Source: CAD feature listing. Evaluate the final solid. Frame: model axes, mm. Give positions to 0.01 mm unless a question says otherwise; leave off trailing zeros. Write each loop counter-clockwise with the first axis right and the second up, starting at its lowest first coordinate (ties: lowest second). Pieces come first, ordered by that corner, then holes. Notation, with made-up numbers: (83, 31.5) -> (104, 31.5) arc R9 cw to (104, 43.5) -> close; hole circle Ø2 at (17.5, -30). An arc over 180 degrees is marked (long way). Answer as a JSON object with one key per item and string values. Group by question number.
Item 1: Ray query, probe 1 along Y at (x, z) = (12.75, 1.45); probe 2 along X at (y, z) = (-2.5, 0.7); probe 3 along Y at (x, z) = (11.25, 2). Return the intervals inside material, ascending. Write a range as from..to.
Item 2: Section query C-C on x = 12.25. Return the cut outline in (y, z), plus the area to 3 significant figures.
Item 3: Section query A-A on z = 0.75. Return the cut outline in (x, y), plus the area to 3 significant figures.
Item 4: First-contact query: pin 1 Ø6 at (x, y) = (7, -2.5) entering from -Z; pin 2 Ø1.5 at (x, z) = (17.5, 1.5) entering from +Y. Flat tips, straight axial feed; report the tip coordinate or a pass-through.
Item 5: Section query B-B on y = -5. Return the cut outline in (x, z), plus the area to 3 significant figures.
Autodesk Inventor part; units mm, degrees
ref_plane "YZ Plane" through (0, 0, 0) normal (1, 0, 0) x (0, 1, 0)
ref_plane "XZ Plane" through (0, 0, 0) normal (0, 1, 0) x (-1, 0, 0)
ref_plane "XY Plane" through (0, 0, 0) normal (0, 0, 1) x (1, 0, 0)
sketch "草图2" plane through (0, 0, 0) normal (0, 0, 1) x (1, 0, 0)
  arc A0 (11.812, -10.0858) -> (14.4114, -9.0466) centre (12.5814, -8.2397) ccw
  arc A1 (11.812, -10.0858) -> (-0.838, -5.8193) centre (-25.1186, -98.698) ccw
  arc A2 (-3.01, -2.276) -> (-0.838, -5.8193) centre (-0.0792, -2.9169) ccw
  line L0 (-0.4446, 9.4555) -> (-3.01, -2.276)
  arc A3 (3.2323, 11.7204) -> (-0.4446, 9.4555) centre (2.4862, 8.8147) ccw
  arc A4 (19.0048, 6.4168) -> (3.2323, 11.7204) centre (-25.1186, -98.698) ccw
  arc A5 (20.0607, 3.7658) -> (19.0048, 6.4168) centre (18.2307, 4.5727) ccw
  line L1 (14.4114, -9.0466) -> (20.0607, 3.7658)
  arc A6 (19.9692, 3.8061) -> (18.9661, 6.3246) centre (18.2307, 4.5727) ccw
  arc A7 (18.9661, 6.3246) -> (3.2074, 11.6235) centre (-25.1186, -98.698) ccw
  arc A8 (3.2074, 11.6235) -> (-0.3469, 9.4342) centre (2.4862, 8.8147) ccw
  line L2 (-0.3469, 9.4342) -> (-2.9123, -2.2974)
  arc A9 (-2.9123, -2.2974) -> (-0.8127, -5.7226) centre (-0.0792, -2.9169) ccw
  arc A10 (11.8505, -9.9935) -> (-0.8127, -5.7226) centre (-25.1186, -98.698) ccw
  arc A11 (11.8505, -9.9935) -> (14.3199, -9.0062) centre (12.5814, -8.2397) ccw
  line L3 (14.3199, -9.0062) -> (19.9692, 3.8061)
  dimension "d2" = 0.1
extrude "拉伸1" add sketch "草图2" along normal blind 3 contours L3 A11 A10 A9 L2 A8 A7 A6
properties part number "斜板固定件"
Worked answers:
{
 "1": {"probe 1": "-10.13..8.72", "probe 2": "-2.95..17.19", "probe 3": "-9.75..9.24"},
 "2": {"outline": "(-10.11, 0) -> (8.9, 0) -> (8.9, 3) -> (-10.11, 3) -> close", "area": "57.0 mm^2"},
 "3": {"outline": "(-2.91, -2.3) arc R2.9 ccw to (-0.81, -5.72) arc R96.1 cw to (11.85, -9.99) arc R1.9 ccw to (14.32, -9.01) -> (19.97, 3.81) arc R1.9 ccw to (18.97, 6.32) arc R113.89 ccw to (3.21, 11.62) arc R2.9 ccw to (-0.35, 9.43) -> close", "area": "347 mm^2"},
 "4": {"pin 1": "z = 0", "pin 2": "y = 7.23"},
 "5": {"outline": "(-2.1, 0) -> (16.09, 0) -> (16.09, 3) -> (-2.1, 3) -> close", "area": "54.5 mm^2"}
}
